The figure shows three views and two pictorial views of one solid part (mm, origin at its lowest corner). Answer the questions. A direction names the side the tool comes from. Coordinates: 2 decimals unless noted, no trailing zeros. Order: outer loops, then holes, each group sorted by start corner. A loop starts at its lowest first (then second) coordinate and runs counter-clockwise, first axis right, second up. Notation, with made-up numbers: (55, 29) -> (70, 29) arc R21 ccw to (70, 49) -> close; hole circle Ø7 at (35.5, -17.5). An arc over 180 degrees is marked (long way). Write item = value, one per line.
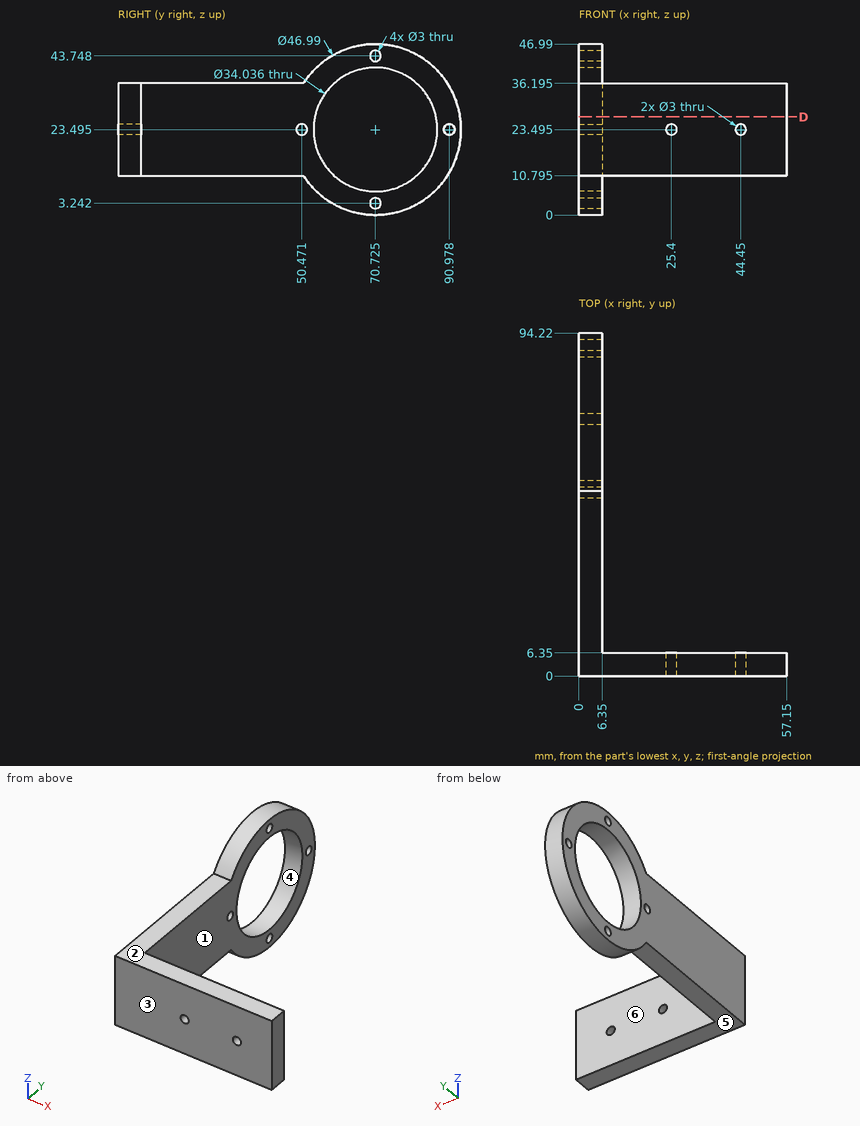
Q1. Each of these flat-tipped pins is pushed along its axis until it touches: pin 1 Ø1 at (x, z) = (47.5, 13) entering from -Y; pin 2 Ø5 at (y, z) = (50.47, 23.5) entering from +X; pin 3 Ø7.5 at (x, z) = (43, 29) entering from +Y. Where does it stop, or does it pass through?
The answers:
pin_1 = 0
pin_2 = 6.35
pin_3 = 6.35
Q2. A tool of negligible diameter and unlimited length cuts with its end or side. For the marked faces 1, 2 and 3, from which of +Z, -Z, +X, -X, +Y, -Y can it reach the whole face along a straight path? Write none if from no direction.
The answers:
face_1 = +Z, -Z, +X, +Y
face_2 = +Z, +X, -X, -Y
face_3 = +Z, -Z, +X, -X, -Y
Q3. Find the intervals of material crossed by line 1 along X through (y, z) = (40, 28); line 2 along Y through (x, z) = (6, 30), in increasing order.
The answers:
line_1 = 0 to 6.35
line_2 = 0 to 55, 86.45 to 93.3
Q4. Section D-D, the plane z = 27 is taken. Give the vertices of the cut face in (x, y).
The answers:
outline = (0, 0) -> (57.15, 0) -> (57.15, 6.35) -> (6.35, 6.35) -> (6.35, 54.07) -> (0, 54.07) -> close; (0, 87.38) -> (6.35, 87.38) -> (6.35, 93.96) -> (0, 93.96) -> close
Q5. The mould has two halves that part along Z. Classify the marked faces 4, 5 and 6: released by +Z, released by -Z, zero draft, split by the parting line, or undercut.
The answers:
face_4 = undercut
face_5 = released by -Z
face_6 = zero draft
